Can you work these out from the model? Positions are in its coordinate system, mm. A direction names the side the tool comes from. Round coordinates to 2 decimals unless told otherwise and drop trailing zeros. Loops run counter-clockwise (first coordinate to the right, second up) from the corner with the lowest first, then second, coordinate; pieces in that order, holes last. Notation, with made-up numbers: (66, 29) -> (72, 29) arc R27 ccw to (72, 55) -> close; hole circle Ø7 at (21.25, -19.75). An arc over 180 degrees is marked (long way). Use a Markdown table: item, result.
from build123d import *

# Parameters (mm, degrees)
EXTRUDE_1_DEPTH      = 19
EXTRUDE_1_DEPTH_BACK = 21
SKETCH_1_R           = 6
SKETCH_3_R           = 3.1
CUT_EXTRUDE_1_DEPTH  = 17
SKETCH_4_R           = 4.1
CUT_EXTRUDE_2_DEPTH  = 21
EXTRUDE_START        = 12
EXTRUDE_2_DEPTH      = 12
EXTRUDE_START_2      = 15
EXTRUDE_3_DEPTH      = 15
CHAMFER_1_SIZE       = 0.4
CHAMFER_2_SIZE       = 0.5


with BuildPart() as part:
    # 草图1 → 凸台-拉伸1 (new, two sides: drawn at the far end of the back side and taken through both)
    with BuildSketch(Plane(origin=(0, 0, 0), x_dir=(0, 0, -1), z_dir=(1, 0, 0)).offset(-EXTRUDE_1_DEPTH_BACK)):
        Circle(SKETCH_1_R)
    extrude(amount=EXTRUDE_1_DEPTH + EXTRUDE_1_DEPTH_BACK)

    # 草图3 → 切除-拉伸1 (cut)
    with BuildSketch(Plane(origin=(19, 0, 0), x_dir=(0, 0, -1), z_dir=(1, 0, 0))):
        Circle(SKETCH_3_R)
    extrude(amount=-CUT_EXTRUDE_1_DEPTH, mode=Mode.SUBTRACT)

    # 草图4 → 切除-拉伸2 (cut)
    with BuildSketch(Plane.ZY.offset(21)):
        Circle(SKETCH_4_R)
    extrude(amount=-CUT_EXTRUDE_2_DEPTH, mode=Mode.SUBTRACT)

    # 草图5 → 凸台-拉伸2 (add)
    with BuildSketch(Plane(origin=(2, 0, 0), x_dir=(0, 0, -1), z_dir=(1, 0, 0)).offset(EXTRUDE_START)):
        with BuildLine():
            Line((-1.688194302, 2.6), (1.688194302, 2.6))
            ThreePointArc((1.688194302, 2.6), (0, 3.1), (-1.688194302, 2.6))
        make_face()
    extrude(amount=-EXTRUDE_2_DEPTH)

    # 草图6 → 凸台-拉伸3 (add)
    with BuildSketch(Plane.ZY.offset(EXTRUDE_START_2)):
        with BuildLine():
            Line((-1.748205844, 3.708608408), (2.169358352, 3.479063716))
            ThreePointArc((2.169358352, 3.479063716), (0.239822956, 4.09297996), (-1.748205844, 3.708608408))
        make_face()
    extrude(amount=-EXTRUDE_3_DEPTH)

    # 倒角1
    chamfer_1_edges = [part.edges().sort_by_distance(p)[0] for p in [
        (-21, 0, -4.1),
        (19, 0, 3.1),
    ]]
    chamfer(chamfer_1_edges, length=CHAMFER_1_SIZE)

    # 倒角2
    chamfer_2_edges = [part.edges().sort_by_distance(p)[0] for p in [
        (-15, 3.593836062, 0.210576254),
        (14, 2.6, 0),
    ]]
    chamfer(chamfer_2_edges, length=CHAMFER_2_SIZE - 0.0001)  # a hair under: the kernel refuses the full size


solid = part.part
1. I need wall thicknesses on line 1 (Y direction, x = 14.5, z = 0); line 2 (Y direction, x = 13.5, z = 0); line 3 (X direction, y = 0, z = -1.75). Which ranges of each line are inside material? Lowest first, please.
Answer sheet:
| item | result |
|---|---|
| line 1 | y = -6 to -3.1, 3.1 to 6 |
| line 2 | y = -6 to -3.1, 2.6 to 6 |
| line 3 | x = 0 to 2 |
2. If we mould it in two halves opening along Y, with no side actions, what happens to faces 4 (the flat face through (-21, 4.5, 1.4)), 5 (the cylindrical face through (-1, 0, 6)), 6 (the cylindrical face through (10.416, -3.026, 0.672))? For each: +Y half, -Y half, draft (parallel to the pull), parting line (faces both ways), or undercut.
Answer sheet:
| item | result |
|---|---|
| face 4 | draft |
| face 5 | parting line |
| face 6 | undercut |
3. Will these pins go through, and if not, where does the flat tip stop? pin 1 Ø2.5 at (y, z) = (-1, 1.5) entering from -X; pin 2 Ø2 at (x, z) = (-9.5, -3.5) entering from +Y; pin 3 Ø5 at (y, z) = (0, 0) entering from +X.
Answer sheet:
| item | result |
|---|---|
| pin 1 | stops at x = 0 |
| pin 2 | stops at y = 5.45 |
| pin 3 | stops at x = 2 |
4. Which directions (+Z, -Z, +X, -X, +Y, -Y) give clear straight access to the entire face, cutting with the end or side of a thin tool? Please do faces 1 (the flat face through (2, 0, 0)), 2 (the cylindrical face through (-10.4, -4, -0.9)), 3 (the flat face through (19, -3, -3)).
Answer sheet:
| item | result |
|---|---|
| face 1 | +X |
| face 2 | -X |
| face 3 | +Z, -Z, +X, +Y, -Y |
5. I want a section at A-A (y = 0). Please give me the cut outline in (x, z).
Answer sheet:
| item | result |
|---|---|
| outline | (-21, -6) -> (19, -6) -> (19, -3.5) -> (18.6, -3.1) -> (2, -3.1) -> (2, 3.1) -> (18.6, 3.1) -> (19, 3.5) -> (19, 6) -> (-21, 6) -> (-21, 4.5) -> (-20.6, 4.1) -> (0, 4.1) -> (0, -4.1) -> (-20.6, -4.1) -> (-21, -4.5) -> close |
6. I want a section at C-C (z = 5.25). Please give me the cut outline in (x, y).
Answer sheet:
| item | result |
|---|---|
| outline | (-21, -2.9) -> (19, -2.9) -> (19, 2.9) -> (-21, 2.9) -> close |
7. I want a section at B-B (x = 9). Please give me the cut outline in (y, z), plus the area to 3 significant figures.
Answer sheet:
| item | result |
|---|---|
| outline | circle Ø12 at (0, 0); hole (2.6, -1.69) -> (2.6, 1.69) arc R3.1 ccw (long way) to start |
| area | 84.1 mm² |
8. I want a section at D-D (y = -5). Please give me the cut outline in (x, z), plus the area to 3 significant figures.
Answer sheet:
| item | result |
|---|---|
| outline | (-21, -3.32) -> (19, -3.32) -> (19, 3.32) -> (-21, 3.32) -> close |
| area | 265 mm² |
